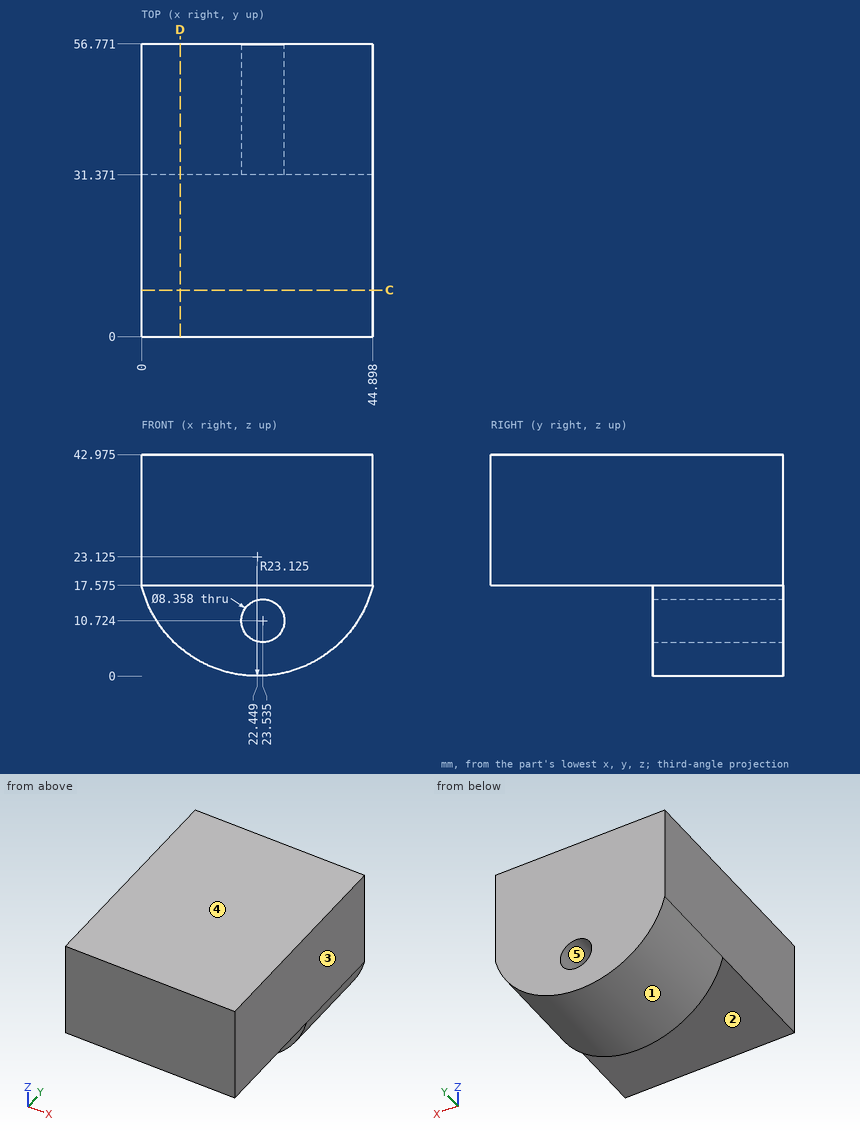
Input: dimensioned drawing with shaded views. Units: mm. Origin: part minimum x, y, z. A direction names the side the tool comes from. Give positions to 0.01 mm unless a question says otherwise; leave off trailing zeros. Order: outer loops, then holes, each group sorted by start corner. A loop starts at its lowest first (then second) coordinate and runs counter-clockwise, first axis right, second up.
(1) Contact query for flat-ended pins moving along their axis: P1, Ø1.5, axis at x = 33, y = 17, coming from the -Z side (1 decimal); P2, Ø5, axis at x = 23.53, z = 10.72, coming from the +Y side; P3, Ø10, axis at x = 17, z = 15, coming from the -Y side. Output: stop coordinate, or through.
(2) Access query for the marked faces 1 and 2. Directions: +Z, -Z, +X, -X, +Y, -Y. A direction counts if a zero-diameter tool reaches every point of the face in a straight line with its end or side. Return the directions, or none.
(3) Pull-direction query (Z, two-part tool) for the marked faces 3, 4 and 5; classes: +Z half, -Z half, draft (parallel to the pull), parting line (faces both ways), or undercut.
(4) Section query C-C (y = 9). Return the cut outline in (x, z) (1 decimal), plus the area to 3 significant figures.
(5) Material intervals for line 1 along Y through (x, z) = (27, 16); line 2 along Z through (x, y) = (26, 25) (1 decimal); line 3 along Z through (x, y) = (23, 32) (1 decimal), sorted ascending.
(6) Section query D-D (x = 7.5). Return the cut outline in (y, z) (1 decimal), plus the area to 3 significant figures.
Outcome:
1. P1: stops at z = 17.6
1. P2: passes through
1. P3: stops at y = 0
2. face 1: -Z, +Y, -Y
2. face 2: -Z, +X, -X, -Y
3. face 3: draft
3. face 4: +Z half
3. face 5: undercut
4. outline: (0, 17.6) - (44.9, 17.6) - (44.9, 43) - (0, 43) - close
4. area: 1,140 mm2
5. line 1: y = 31.37 to 56.77
5. line 2: z = 17.6 to 43
5. line 3: z = 0 to 6.6, 14.9 to 43
6. outline: (0, 17.6) - (31.4, 17.6) - (31.4, 5.5) - (56.8, 5.5) - (56.8, 43) - (0, 43) - close
6. area: 1,750 mm2
